For this review, use the dimensioned drawing (mm, ordinates from the lowest corner) and the shaded views. A direction names the side the tool comes from. Coordinates: 2 decimals unless noted, no trailing zeros. Loops run counter-clockwise (first coordinate to the right, second up) from the corner with the lowest first, then second, coordinate; pieces in that order, holes last. Notation, with made-up numbers: (66.25, -20.5) -> (111.25, -20.5) arc R28 ccw to (111.25, 17.5) -> close; hole circle Ø9 at (10.5, 38.25). An arc over 180 degrees is marked (long way). Use one line per item in the form item = value. Start each with the question number.
1. Consider section A-A (x = 61). State the section outline as (y, z) points.
2. Consider section C-C (y = 12). State the section outline as (x, z) points.
3. For pin 1 (7.5 mm diameter, centred on x = 87, y = 10, fed in from -Z); pin 2 (20 mm diameter, centred on x = 84.5, y = 32.5, fed in from -Z); pin 3 (4.5 mm diameter, centred on x = 17, y = 10.5, fed in from +Z), all flat-tipped, find the tip position at first contact; note any pin that passes through.
4. The part is to be moulded in two halves that separate along X. For the marked faces 1, 2, 3 and 4, say which applies: released by +X, released by -X, zero draft, split by the parting line, or undercut.
5. Machinability: for the marked faces 5, 6 and 7, which of the approach directions +Z, -Z, +X, -X, +Y, -Y give a long, thin tool a straight path to every point of the face, cutting with its end or side? Answer none if there is none.
6. Consider section D-D (z = 5). State the section outline as (x, y) points.
7. Consider section B-B (y = 26). State the section outline as (x, z) points.
8. Wall thickness on line 1 (Z direction, x = 56, y = 7); line 2 (X direction, y = 8, z = 26.5); line 3 (Z direction, x = 81.5, y = 7): over which ranges is each line inside the solid? List them lowest first. Write a range as from..to.
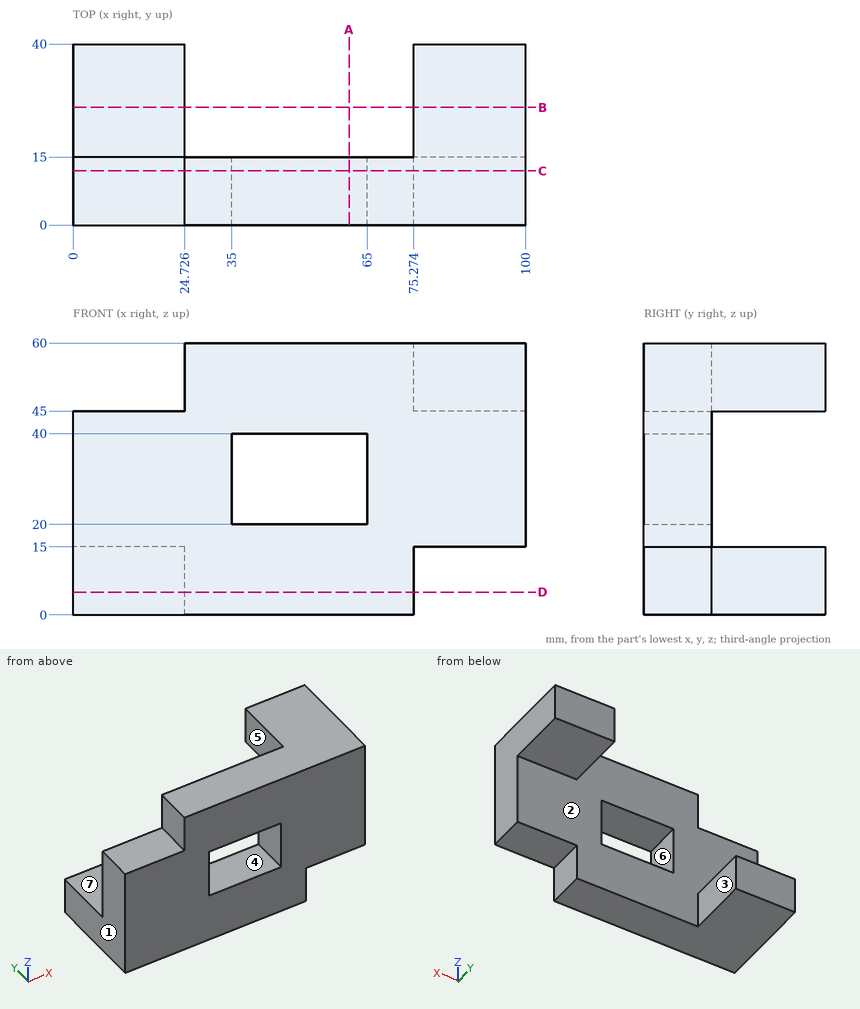
Geometry check:
q1.outline = (0, 0) -> (15, 0) -> (15, 20) -> (0, 20) -> close; (0, 40) -> (15, 40) -> (15, 60) -> (0, 60) -> close
q2.outline = (0, 0) -> (75.27, 0) -> (75.27, 15) -> (100, 15) -> (100, 60) -> (24.73, 60) -> (24.73, 45) -> (0, 45) -> close; hole (35, 20) -> (65, 20) -> (65, 40) -> (35, 40) -> close
q3.pin_1 = 15
q3.pin_2 = 45
q3.pin_3 = 45
q4.face_1 = released by -X
q4.face_2 = zero draft
q4.face_3 = released by +X
q4.face_4 = undercut
q5.face_5 = +Z, -Z, -X, +Y
q5.face_6 = +Y, -Y
q5.face_7 = +Z, +X, -X, +Y
q6.outline = (0, 0) -> (75.27, 0) -> (75.27, 15) -> (24.73, 15) -> (24.73, 40) -> (0, 40) -> close
q7.outline = (0, 0) -> (24.73, 0) -> (24.73, 15) -> (0, 15) -> close; (75.27, 45) -> (100, 45) -> (100, 60) -> (75.27, 60) -> close
q8.line_1 = 0..20, 40..60
q8.line_2 = 0..35, 65..100
q8.line_3 = 15..60
